Input: part model. Units: mm. Frame: model coordinates. Coordinates: 2 decimals unless noted, no trailing zeros. Write each loop counter-clockwise with the first axis right and the second up, starting at its lowest first coordinate (ties: lowest second). Pieces come first, ordered by that corner, then holes. Notation, with made-up numbers: (-10.75, -24.75) - (23.25, -24.75) arc R13 ccw to (23.25, -4.75) - close; hole circle Ø4 at (27, 43.5). An arc over 180 degrees is marked (long way). One line per question, with ' | ' between items. Start each with the question number.
1) Section query A-A on z = 0.9. Return loops of the section in (x, y), and give its area (3 significant figures).
2) Section query C-C on x = -9. Return loops of the section in (y, z).
3) Section query D-D on y = 18. Return loops of the section in (x, z), and give its area (3 significant figures).
4) First-contact query: P1, Ø10, axis at x = -15.5, y = 5, coming from the -Z side; P2, Ø0.8, axis at x = 2, z = 0.5, coming from the +Y side. Flat tips, straight axial feed; report the tip coordinate or a pass-through.
5) Line query: line 1 (X direction, y = -1, z = 1.35); line 2 (X direction, y = 11, z = 0.6); line 3 (Y direction, x = -18, z = 0.7). Output: solid intervals per line, ascending.
6) Section query B-B on y = -8.5. Return loops of the section in (x, z).
```python
from build123d import *

# Parameters (mm, degrees)
F1_DEPTH = 1.5


with BuildPart() as f1:
    # F0 (on Top) → F1 (new body)
    with BuildSketch(Plane.XY):
        with BuildLine():
            ThreePointArc((24.345579, -21.095447), (28.363111, -19.224056), (30, -15.105408))
            Line((30, -15.105408), (30, 15.105408))
            ThreePointArc((30, 15.105408), (28.363111, 19.224056), (24.345579, 21.095447))
            Line((24.345579, 21.095447), (0, 22.5))
            Line((0, 22.5), (-24.345579, 21.095447))
            ThreePointArc((-24.345579, 21.095447), (-28.363111, 19.224056), (-30, 15.105408))
            Line((-30, 15.105408), (-30, -15.105408))
            ThreePointArc((-30, -15.105408), (-28.363111, -19.224056), (-24.345579, -21.095447))
            Line((-24.345579, -21.095447), (0, -22.5))
            Line((0, -22.5), (24.345579, -21.095447))
        make_face()
        with BuildLine():
            ThreePointArc((24, -0.5), (19.167262, -12.167262), (7.5, -17))
            Line((7.5, -17), (-7.4, -17))
            ThreePointArc((-7.4, -17), (-19.137973, -12.137973), (-24, -0.4))
            Line((-24, -0.4), (-24, 0.5))
            ThreePointArc((-24, 0.5), (-19.167262, 12.167262), (-7.5, 17))
            Line((-7.5, 17), (7.5, 17))
            ThreePointArc((7.5, 17), (19.167262, 12.167262), (24, 0.5))
            Line((24, 0.5), (24, -0.5))
        make_face(mode=Mode.SUBTRACT)
    extrude(amount=F1_DEPTH)


solid = f1.part
```
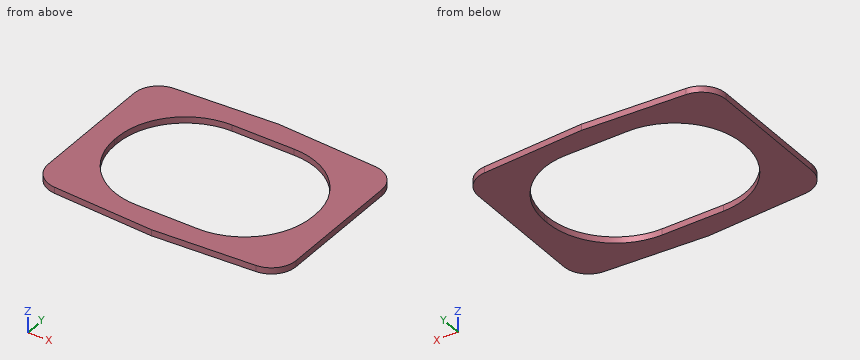
Answer key:
1) outline: (-30, -15.11) arc R6 ccw to (-24.35, -21.1) - (0, -22.5) - (24.35, -21.1) arc R6 ccw to (30, -15.11) - (30, 15.11) arc R6 ccw to (24.35, 21.1) - (0, 22.5) - (-24.35, 21.1) arc R6 ccw to (-30, 15.11) - close; hole (-24, -0.4) arc R16.6 ccw to (-7.4, -17) - (7.5, -17) arc R16.5 ccw to (24, -0.5) - (24, 0.5) arc R16.5 ccw to (7.5, 17) - (-7.5, 17) arc R16.5 ccw to (-24, 0.5) - close | area: 1,170 mm²
2) outline: (-21.98, 0) - (-16.92, 0) - (-16.92, 1.5) - (-21.98, 1.5) - close; (16.93, 0) - (21.98, 0) - (21.98, 1.5) - (16.93, 1.5) - close
3) outline: (-29.26, 0) - (29.26, 0) - (29.26, 1.5) - (-29.26, 1.5) - close | area: 87.8 mm²
4) P1: through | P2: y = 22.41
5) line 1: -30 to -23.99, 23.99 to 30 | line 2: -30 to -20.23, 20.23 to 30 | line 3: -21.46 to -13.17, 13.23 to 21.46
6) outline: (-30, 0) - (-21.89, 0) - (-21.89, 1.5) - (-30, 1.5) - close; (21.93, 0) - (30, 0) - (30, 1.5) - (21.93, 1.5) - close
